from build123d import *
from OCP.BRepFilletAPI import BRepFilletAPI_MakeChamfer

# Parameters (mm, degrees)
SKETCH1_W           = 76.2
SKETCH1_H           = 76.2
SKETCH1_W_2         = 69.85
SKETCH1_H_2         = 69.85
BOSS_EXTRUDE1_DEPTH = 9.525
SKETCH2_R           = 1.26365
CUT_EXTRUDE1_DEPTH  = 86.725
CHAMFER1_SIZE       = 2.54
CHAMFER1_SIZE2      = 2.207988314
SKETCH3_W           = 76.2
SKETCH3_H           = 76.2
SKETCH3_W_2         = 69.85
SKETCH3_H_2         = 69.85
BOSS_EXTRUDE2_DEPTH = 139.7


with BuildPart() as part:
    # Sketch1 → Boss-Extrude1 (new body)
    with BuildSketch(Plane(origin=(0, 0, 0), x_dir=(1, 0, 0), z_dir=(0, 1, 0))):
        Rectangle(SKETCH1_W, SKETCH1_H)
        Rectangle(SKETCH1_W_2, SKETCH1_H_2, mode=Mode.SUBTRACT)
    extrude(amount=BOSS_EXTRUDE1_DEPTH)

    # Sketch2 → Cut-Extrude1 (cut, through all)
    with BuildSketch(Plane.XY.offset(38.1)):
        with Locations((-12.7, 4.7625)):
            Circle(SKETCH2_R)
        with Locations((12.7, 4.7625)):
            Circle(SKETCH2_R)
    extrude(amount=-CUT_EXTRUDE1_DEPTH, mode=Mode.SUBTRACT)

    # Chamfer1: one chamfer whose edges measure the first distance from different faces: ONE call of the kernel's chamfer builder (chamfer() names one face for all edges)
    chamfer1_edges_1 = [part.edges().sort_by_distance(p)[0] for p in [
        (-13.96365, 4.7625, -38.1),
    ]]
    chamfer1_side_1 = [part.faces().sort_by_distance(p)[0] for p in [
        (-13.96365, 4.7625, -36.5125),
    ]]
    chamfer1_edges_2 = [part.edges().sort_by_distance(p)[0] for p in [
        (-13.96365, 4.7625, 38.1),
        (11.43635, 4.7625, 38.1),
    ]]
    chamfer1_side_2 = [part.faces().sort_by_distance(p)[0] for p in [
        (0, 4.7625, 38.1),
    ]]
    chamfer1_edges_3 = [part.edges().sort_by_distance(p)[0] for p in [
        (11.43635, 4.7625, -38.1),
    ]]
    chamfer1_side_3 = [part.faces().sort_by_distance(p)[0] for p in [
        (11.43635, 4.7625, -36.5125),
    ]]
    chamfer1 = BRepFilletAPI_MakeChamfer(part.part.solid().wrapped)
    for e in chamfer1_edges_1:
        chamfer1.Add(CHAMFER1_SIZE, CHAMFER1_SIZE2, e.wrapped, chamfer1_side_1[0].wrapped)  # the first distance lies on this face
    for e in chamfer1_edges_2:
        chamfer1.Add(CHAMFER1_SIZE, CHAMFER1_SIZE2, e.wrapped, chamfer1_side_2[0].wrapped)  # the first distance lies on this face
    for e in chamfer1_edges_3:
        chamfer1.Add(CHAMFER1_SIZE, CHAMFER1_SIZE2, e.wrapped, chamfer1_side_3[0].wrapped)  # the first distance lies on this face
    add(Compound.cast(chamfer1.Shape()), mode=Mode.REPLACE)

    # Sketch3 → Boss-Extrude2 (add)
    with BuildSketch(Plane(origin=(0, 9.525, 0), x_dir=(1, 0, 0), z_dir=(0, 1, 0))):
        Rectangle(SKETCH3_W, SKETCH3_H)
        Rectangle(SKETCH3_W_2, SKETCH3_H_2, mode=Mode.SUBTRACT)
    extrude(amount=BOSS_EXTRUDE2_DEPTH)


solid = part.part
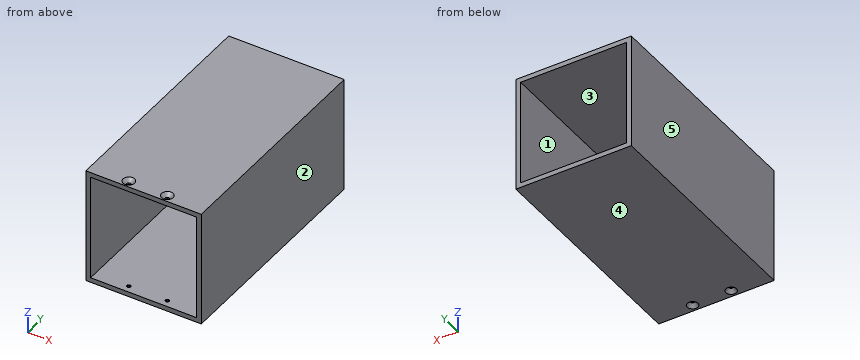
Can you work these out from the model? Positions are in its coordinate system, mm. Face numbers are marked on the shaded views. A direction names the side the tool comes from. Coordinates: 2 decimals unless noted, no trailing zeros. Write each loop counter-clockwise with the first axis right and the second up, starting at its lowest first coordinate (ties: lowest second). Pieces come first, ordered by that corner, then holes.
Q1. Imagine slicing it at A-A, the plane y = 43. List the corners of the cut face in (x, z) for me (3 decimals).
Results found:
outline: (-38.1, -38.1) - (38.1, -38.1) - (38.1, 38.1) - (-38.1, 38.1) - close; hole (-34.925, -34.925) - (34.925, -34.925) - (34.925, 34.925) - (-34.925, 34.925) - close
Q2. Imagine slicing it at C-C, the plane x = -18.5. List the corners of the cut face in (y, z) for me (3 decimals).
Results found:
outline: (0, -38.1) - (149.225, -38.1) - (149.225, -34.925) - (0, -34.925) - close; (0, 34.925) - (149.225, 34.925) - (149.225, 38.1) - (0, 38.1) - close
Q3. Please list where these lines run through material, in increasing order: L1, parallel to Y at x = 12.7, z = -35.15 (3 decimals); L2, parallel to X at y = 65, z = 25 (3 decimals).
Results found:
L1: y = 0 to 3.499, 6.026 to 149.225
L2: x = -38.1 to -34.925, 34.925 to 38.1
Q4. If we mould it in two halves opening along X, with no side actions, what happens to the marked faces 3, 4 and 5? For each: +X half, -X half, draft (parallel to the pull), parting line (faces both ways), or undercut.
Results found:
face 3: undercut
face 4: draft
face 5: -X half
Q5. Which directions (+Z, -Z, +X, -X, +Y, -Y) give clear straight access to the entire face, cutting with the end or side of a thin tool? Please do the marked faces 1 and 2.
Results found:
face 1: +Y, -Y
face 2: +Z, -Z, +X, +Y, -Y
Q6. Imagine slicing it at B-B, the plane z = 10.5. List the corners of the cut face in (x, y) for me (3 decimals), plus the area to 3 significant figures.
Results found:
outline: (-38.1, 0) - (-34.925, 0) - (-34.925, 149.225) - (-38.1, 149.225) - close; (34.925, 0) - (38.1, 0) - (38.1, 149.225) - (34.925, 149.225) - close
area: 948 mm2
